from build123d import *

# Parameters (mm, degrees)
BOSS_EXTRUDE1_DEPTH = 1
SKETCH2_R           = 1
BOSS_EXTRUDE2_DEPTH = 1
FILLET1_R           = 3
CUT_EXTRUDE1_REACH  = 3
SKETCH3_R           = 1.55


with BuildPart() as part:
    # Sketch1 → Boss-Extrude1 (new body)
    with BuildSketch(Plane.XY):
        Polygon((-8, 5), (-8, 38), (-59.580513121, 38), (-59.580513121, 27.2), (-41, 27.2), (-41, 5), align=None)
    extrude(amount=BOSS_EXTRUDE1_DEPTH)

    # Sketch2 → Boss-Extrude2 (add)
    with BuildSketch(Plane.XY.offset(1)):
        with Locations((-12, 9)):
            Circle(SKETCH2_R)
        with Locations((-12, 13.3)):
            Circle(SKETCH2_R)
        with Locations((-12, 17.6)):
            Circle(SKETCH2_R)
        with Locations((-12, 21.9)):
            Circle(SKETCH2_R)
        with Locations((-12, 26.2)):
            Circle(SKETCH2_R)
        with Locations((-12, 30.5)):
            Circle(SKETCH2_R)
        with Locations((-12, 34.8)):
            Circle(SKETCH2_R)
        with Locations((-16.3, 9)):
            Circle(SKETCH2_R)
        with Locations((-20.6, 9)):
            Circle(SKETCH2_R)
        with Locations((-24.9, 9)):
            Circle(SKETCH2_R)
        with Locations((-29.2, 9)):
            Circle(SKETCH2_R)
        with Locations((-33.5, 9)):
            Circle(SKETCH2_R)
        with Locations((-37.8, 9)):
            Circle(SKETCH2_R)
        with Locations((-16.3, 34.8)):
            Circle(SKETCH2_R)
        with Locations((-20.6, 34.8)):
            Circle(SKETCH2_R)
        with Locations((-24.9, 34.8)):
            Circle(SKETCH2_R)
        with Locations((-29.2, 34.8)):
            Circle(SKETCH2_R)
        with Locations((-33.5, 34.8)):
            Circle(SKETCH2_R)
        with Locations((-37.8, 34.8)):
            Circle(SKETCH2_R)
        with Locations((-42.1, 34.8)):
            Circle(SKETCH2_R)
        with Locations((-46.4, 34.8)):
            Circle(SKETCH2_R)
        with Locations((-50.7, 34.8)):
            Circle(SKETCH2_R)
        with Locations((-55, 34.8)):
            Circle(SKETCH2_R)
        with BuildLine():
            Line((-35.8, 30.5), (-18.3, 30.5))
            ThreePointArc((-18.3, 30.5), (-16.885786438, 29.914213562), (-16.3, 28.5))
            Line((-16.3, 28.5), (-16.3, 15.236025644))
            ThreePointArc((-16.3, 15.236025644), (-16.885786438, 13.821812082), (-18.3, 13.236025644))
            Line((-18.3, 13.236025644), (-35.8, 13.236025644))
            ThreePointArc((-35.8, 13.236025644), (-37.214213562, 13.821812082), (-37.8, 15.236025644))
            Line((-37.8, 15.236025644), (-37.8, 28.5))
            ThreePointArc((-37.8, 28.5), (-37.214213562, 29.914213562), (-35.8, 30.5))
        make_face()
        with BuildLine():
            Line((-35.8, 29.5), (-18.3, 29.5))
            ThreePointArc((-18.3, 29.5), (-17.592893219, 29.207106781), (-17.3, 28.5))
            Line((-17.3, 28.5), (-17.3, 15.236025644))
            ThreePointArc((-17.3, 15.236025644), (-17.592893219, 14.528918863), (-18.3, 14.236025644))
            Line((-18.3, 14.236025644), (-35.8, 14.236025644))
            ThreePointArc((-35.8, 14.236025644), (-36.507106781, 14.528918863), (-36.8, 15.236025644))
            Line((-36.8, 15.236025644), (-36.8, 28.5))
            ThreePointArc((-36.8, 28.5), (-36.507106781, 29.207106781), (-35.8, 29.5))
        make_face(mode=Mode.SUBTRACT)
    extrude(amount=BOSS_EXTRUDE2_DEPTH)

    # Fillet1
    fillet1_edges = [part.edges().sort_by_distance(p)[0] for p in [
        (-41, 5, 0.5),
        (-41, 27.2, 0.5),
        (-59.580513121, 27.2, 0.5),
        (-59.580513121, 38, 0.5),
        (-8, 38, 0.5),
        (-8, 5, 0.5),
    ]]
    fillet(fillet1_edges, radius=FILLET1_R)

    # Sketch3 → Cut-Extrude1 (cut, up to next)
    with BuildSketch(Plane.XY.offset(1), mode=Mode.PRIVATE) as cut_extrude1_sk1:
        with Locations((-20.677552724, 17.314204089)):
            Circle(SKETCH3_R)
    cut_extrude1_tool1 = extrude(cut_extrude1_sk1.sketch, amount=-CUT_EXTRUDE1_REACH, mode=Mode.PRIVATE) & part.part
    add(cut_extrude1_tool1.solids().sort_by_distance((-20.677553, 17.314204, 1))[0], mode=Mode.SUBTRACT)
    # Sketch3 → Cut-Extrude1 (cut, up to next)
    with BuildSketch(Plane.XY.offset(1), mode=Mode.PRIVATE) as cut_extrude1_sk2:
        with Locations((-55, 30.651276125)):
            Circle(SKETCH3_R)
    cut_extrude1_tool2 = extrude(cut_extrude1_sk2.sketch, amount=-CUT_EXTRUDE1_REACH, mode=Mode.PRIVATE) & part.part
    add(cut_extrude1_tool2.solids().sort_by_distance((-55, 30.651276, 1))[0], mode=Mode.SUBTRACT)


solid = part.part
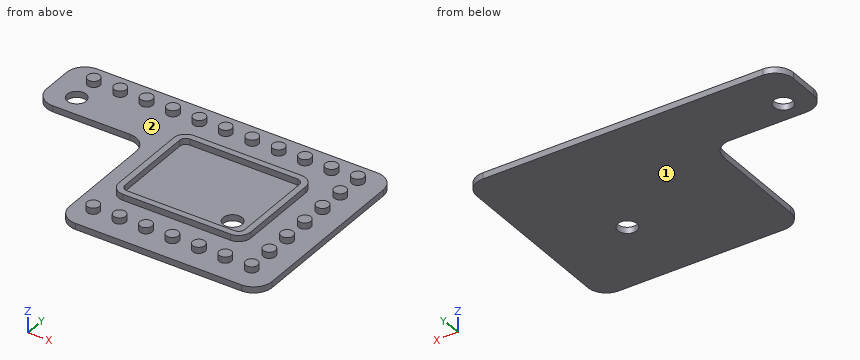
Input: part model. Units: mm. Frame: model coordinates. Face numbers are marked on the shaded views. Give positions to 0.01 mm unless a question says otherwise; leave off trailing zeros. Write each loop counter-clockwise with the first axis right and the second up, starting at its lowest first coordinate (ties: lowest second). Pieces come first, ordered by that corner, then holes. Notation, with made-up numbers: M -17,89.25 L 25,89.25 A32 ccw 25,117.25 Z; hole C 16,-11.75 d1. An arc over 180 degrees is marked long. Use one line per item in the form item = value.
1. Mould query, pull axis Y, two halves, no side actions, for the marked faces 1 and 2. Classes: released by +Y, released by -Y, zero draft, split by the parting line, or undercut.
Outcome:
face_1 = zero draft
face_2 = undercut
2. Cut plane B-B on y = 21.9. Return loops of the section in (x, z).
Outcome:
outline = M -41,0 L -8,0 L -8,1 L -11,1 L -11,2 L -13,2 L -13,1 L -16.3,1 L -16.3,2 L -17.3,2 L -17.3,1 L -36.8,1 L -36.8,2 L -37.8,2 L -37.8,1 L -41,1 Z
3. Cut plane C-C on x = -29.2. Return loops of the section in (y, z).
Outcome:
outline = M 5,0 L 38,0 L 38,1 L 35.8,1 L 35.8,2 L 33.8,2 L 33.8,1 L 30.5,1 L 30.5,2 L 29.5,2 L 29.5,1 L 14.24,1 L 14.24,2 L 13.24,2 L 13.24,1 L 10,1 L 10,2 L 8,2 L 8,1 L 5,1 Z
4. Cut plane D-D on x = -50.5. Return loops of the section in (y, z), and give its area (3 significant figures).
Outcome:
outline = M 27.2,0 L 38,0 L 38,1 L 35.78,1 L 35.78,2 L 33.82,2 L 33.82,1 L 27.2,1 Z
area = 12.8 mm²
5. Cut plane A-A on x = -21. Return loops of the section in (y, z), and give its area (3 significant figures).
Outcome:
outline = M 5,0 L 15.8,0 L 15.8,1 L 14.24,1 L 14.24,2 L 13.24,2 L 13.24,1 L 9.92,1 L 9.92,2 L 8.08,2 L 8.08,1 L 5,1 Z; M 18.83,0 L 38,0 L 38,1 L 35.72,1 L 35.72,2 L 33.88,2 L 33.88,1 L 30.5,1 L 30.5,2 L 29.5,2 L 29.5,1 L 18.83,1 Z
area = 35.6 mm²
6. Ray query, L1, parallel to Y at x = -23, z = 1.8; L2, parallel to X at y = 20, z = 1.55; L3, parallel to Y at x = -55, z = 0.45. Return the intervals inside material, ascending.
Outcome:
L1 = 13.24 to 14.24, 29.5 to 30.5
L2 = -37.8 to -36.8, -17.3 to -16.3
L3 = 27.2 to 29.1, 32.2 to 38
7. First-contact query: P1, Ø0.8, axis at x = -50.5, z = 0.5, coming from the -Y side; P2, Ø0.5, axis at x = -24.5, z = 1.5, coming from the +Y side; P3, Ø3, axis at x = -55, y = 30.65, coming from the -Z side; P4, Ø0.8, axis at y = 12.5, z = 0.5, coming from the -X side. Flat tips, straight axial feed; report the tip coordinate or a pass-through.
Outcome:
P1 = 27.2
P2 = 35.79
P3 = through
P4 = -41
